Design review of the part shown in the three views and the two pictorial views. Dimensions are in mm from the part's minimum x, y and z. A direction names the side the tool comes from. Coordinates: 2 decimals unless noted, no trailing zeros. Write each loop counter-clockwise with the first axis right and the second up, starting at its lowest first coordinate (ties: lowest second). Pieces come first, ordered by that corner, then holes. Notation, with made-up numbers: M 31,41 L 83,41 A23 ccw 83,72 Z; hole C -10,-12.5 d8. An arc over 180 degrees is marked long. Answer as a JSON object with one key per item and string values.
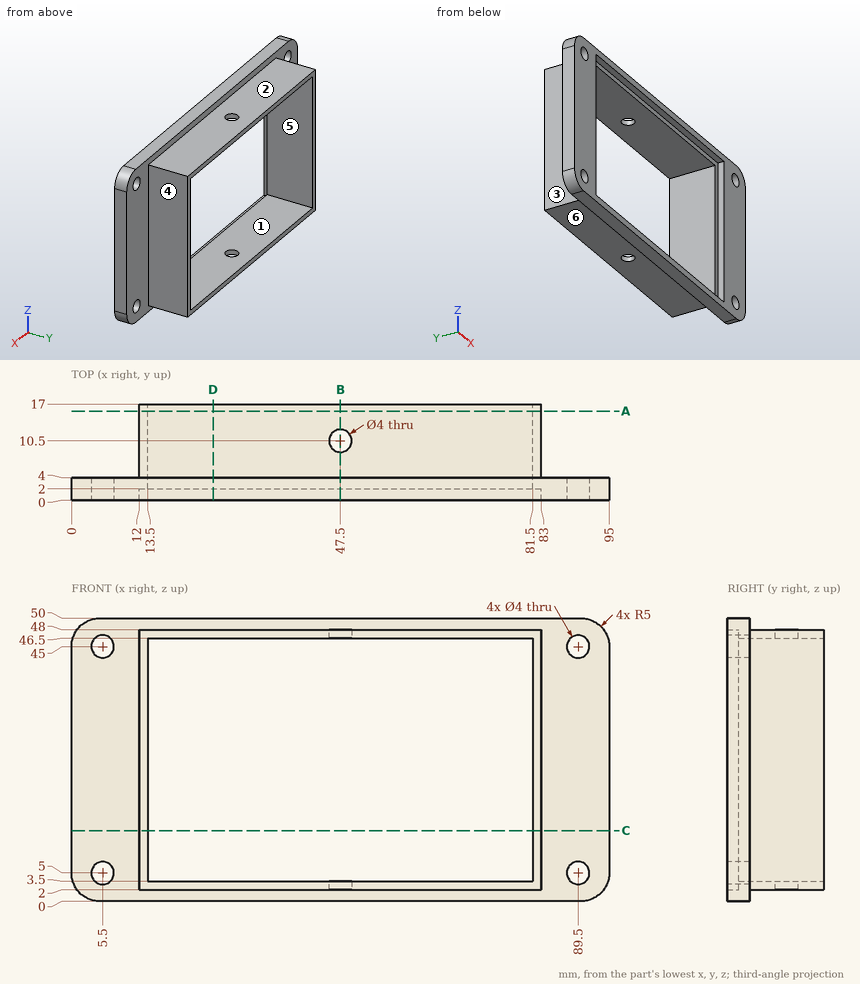
(1) Wall thickness on line 1 along X through (y, z) = (2.65, 5); line 2 along X through (y, z) = (1.4, 45); line 3 along X through (y, z) = (13.25, 12.5): over which ranges is each line inside the solid? List them lowest first. Write a range as from..to.
Results list:
{"line 1": "0..3.5, 7.5..13.5, 81.5..87.5, 91.5..95", "line 2": "0..3.5, 7.5..12, 83..87.5, 91.5..95", "line 3": "12..13.5, 81.5..83"}
(2) For pin 1 Ø4.5 at (y, z) = (7, 20) entering from -X; pin 2 Ø5 at (x, z) = (5.5, 5) entering from +Y; pin 3 Ø4.5 at (x, y) = (47.5, 10.5) entering from -Z, all flat-tipped, find the tip position at first contact; note any pin that passes through.
Results list:
{"pin 1": "x = 12", "pin 2": "y = 4", "pin 3": "z = 2"}
(3) Draft analysis for pull direction X (two halves, no side actions). For the marked faces 4, 5 and 6, state which applies: released by +X, released by -X, zero draft, split by the parting line, or undercut.
Results list:
{"face 4": "released by +X", "face 5": "undercut", "face 6": "zero draft"}
(4) Add section B-B on x = 47.5. Give the boundary of the cut face in (y, z).
Results list:
{"outline": "M 0,0 L 4,0 L 4,2 L 8.5,2 L 8.5,3.5 L 2,3.5 L 2,2 L 0,2 Z; M 0,48 L 2,48 L 2,46.5 L 8.5,46.5 L 8.5,48 L 4,48 L 4,50 L 0,50 Z; M 12.5,2 L 17,2 L 17,3.5 L 12.5,3.5 Z; M 12.5,46.5 L 17,46.5 L 17,48 L 12.5,48 Z"}
(5) For the marked faces 1, 2 and 3, list the 3-axis set-ups (+Z, -Z, +X, -X, +Y, -Y) from which the entire face can be reached by the end or side of a thin tool; tool diameter is ignored.
Results list:
{"face 1": "+Y, -Y", "face 2": "+Z, +X, -X, +Y", "face 3": "+Z, -Z, -X, +Y"}
(6) Add section A-A on y = 15.75. Give the boundary of the cut face in (x, z), and give its area (3 significant figures).
Results list:
{"outline": "M 12,2 L 83,2 L 83,48 L 12,48 Z; hole M 13.5,3.5 L 81.5,3.5 L 81.5,46.5 L 13.5,46.5 Z", "area": "342 mm²"}
(7) Add section D-D on x = 25. Give the boundary of the cut face in (y, z), and give its area (3 significant figures).
Results list:
{"outline": "M 0,0 L 4,0 L 4,2 L 17,2 L 17,3.5 L 2,3.5 L 2,2 L 0,2 Z; M 0,48 L 2,48 L 2,46.5 L 17,46.5 L 17,48 L 4,48 L 4,50 L 0,50 Z", "area": "61.0 mm²"}
(8) Add section C-C on z = 12.5. Give the boundary of the cut face in (x, y).
Results list:
{"outline": "M 0,0 L 12,0 L 12,2 L 13.5,2 L 13.5,17 L 12,17 L 12,4 L 0,4 Z; M 81.5,2 L 83,2 L 83,0 L 95,0 L 95,4 L 83,4 L 83,17 L 81.5,17 Z"}
